```python
from build123d import *

# Parameters (mm, degrees)
SKETCH1_R           = 6.35
BOSS_EXTRUDE1_DEPTH = 31.75
BOSS_EXTRUDE2_DEPTH = 6.35
SKETCH3_R           = 6.35
CUT_EXTRUDE1_DEPTH  = 12.7
FILLET1_R           = 2.54


with BuildPart() as part:
    # Sketch1 → Boss-Extrude1 (new body)
    with BuildSketch(Plane.XY):
        with BuildLine():
            Line((6.565823388424392, 24.536706446302436), (50.800000000000004, 12.699999999999978))
            Line((50.800000000000004, 12.699999999999978), (50.800000000000004, -12.70000000000002))
            Line((50.800000000000004, -12.70000000000002), (6.565823388424392, -24.536706446302436))
            ThreePointArc((6.565823388424392, -24.536706446302436), (-25.400000000000006, 3.11e-15), (6.565823388424392, 24.536706446302436))
        make_face()
        Circle(SKETCH1_R, mode=Mode.SUBTRACT)
    boss_extrude1 = extrude(amount=BOSS_EXTRUDE1_DEPTH)

    # Sketch2 → Boss-Extrude2 (add)
    with BuildSketch(Plane.XY.offset(31.75)):
        with BuildLine():
            Line((50.80000000000001, -12.700000000000014), (50.800000000000004, 12.699999999999978))
            Line((50.800000000000004, 12.699999999999978), (28.910843041272116, 18.557360645652828))
            ThreePointArc((28.910843041272116, 18.557360645652825), (26.285427110394792, 9.443273439243344), (25.399999999999693, 0))
            ThreePointArc((25.399999999999693, 0), (26.285427110394785, -9.443273439243356), (28.910843041272116, -18.557360645652846))
            Line((28.910843041272113, -18.557360645652846), (50.80000000000001, -12.700000000000015))
        make_face()
    boss_extrude2 = extrude(amount=BOSS_EXTRUDE2_DEPTH)

    # Mirror1: Boss-Extrude1, Boss-Extrude2 across plane
    add(boss_extrude1.mirror(Plane.XY))
    add(boss_extrude2.mirror(Plane.XY))

    # Sketch3 → Cut-Extrude1 (cut)
    with BuildSketch(Plane(origin=(50.800000000000004, 0, 0), x_dir=(0, 0, -1), z_dir=(1, 0, 0))):
        Circle(SKETCH3_R)
    extrude(amount=-CUT_EXTRUDE1_DEPTH, mode=Mode.SUBTRACT)

    # Fillet1
    fillet1_edges = [part.edges().sort_by_distance(p)[0] for p in [
        (50.800000000000004, 12.699999999999978, 0),
        (50.80000000000001, -12.700000000000014, 0),
        (17.738333214848257, 21.54703354597763, 31.75),
        (-25.40000000000001, 5.33e-15, 31.75),
        (28.910843041272116, 18.557360645652828, 34.925),
        (28.910843041272116, -18.557360645652842, 34.925),
        (39.85542152063606, 15.628680322826403, 38.1),
        (25.3999999999997, -8.88e-15, 38.1),
        (39.855421520636064, -15.62868032282643, 38.1),
        (17.738333214848254, -21.54703354597764, 31.75),
        (50.80000000000001, -1.776e-14, 38.1),
        (17.738333214848254, -21.54703354597764, -31.75),
        (-25.40000000000001, 5.33e-15, -31.75),
        (17.738333214848257, 21.54703354597763, -31.75),
        (39.85542152063606, 15.628680322826403, -38.1),
        (28.910843041272116, 18.557360645652828, -34.925),
        (50.80000000000001, -1.776e-14, -38.1),
        (39.855421520636064, -15.62868032282643, -38.1),
        (25.3999999999997, -8.88e-15, -38.1),
        (28.910843041272116, -18.557360645652842, -34.925),
    ]]
    fillet(fillet1_edges, radius=FILLET1_R)


solid = part.part
```
CAD build for the part. Positions are in the model's coordinates, mm. A direction names the side the tool comes from. Round coordinates to 2 decimals unless told otherwise and drop trailing zeros. Loops run counter-clockwise (first coordinate to the right, second up) from the corner with the lowest first, then second, coordinate; pieces in that order, holes last. Notation, with made-up numbers: M 38.5,30.25 L 96.5,30.25 A16 ccw 96.5,55.25 Z; hole C 8,36.25 d3. An arc over 180 degrees is marked long. Return JSON: item names as keys, results as strings. Group by question number.
(1) Drop flat-ended pins along their axis: P1, Ø5, axis at y = 11.5, z = -12.5, coming from the -X side; P2, Ø1.5, axis at x = 29.5, z = 5, coming from the -Y side; P3, Ø10, axis at x = -7, y = 19.5, coming from the +Z side. Give the stop position or say it passes through.
(2) Saw through at B-B, the plane z = 0. List the corners of the cut face in (x, y), and give its area (3 significant figures).
(3) Tool access for faces 1 (the cylindrical face through (25.4, 0.2, 33.6)), 2 (the cylindrical face through (29.28, -17.73, -33.14)), 3 (the flat face through (38.1, 0, 0)), 4 (the cylindrical face through (29.28, 17.73, -33.14)): list every direction of +Z, -Z, +X, -X, +Y, -Y with a clear straight run to the whole face (end or side of a thin tool).
(4) Saw through at A-A, the plane x = 0. List the corners of the cut face in (y, z), and give its area (3 significant figures).
(5) Mould opens along Z. For faces 5 (the cylindrical face through (18.8, 20.5, -31)), 6 (the cylindrical face through (18.8, 20.5, 31)), 7 (the cylindrical face through (44.54, -6.2, 1.38)), 8 (the cylindrical face through (50.29, 12.28, 0.5)) say: +Z half, -Z half, draft (parallel to the pull), parting line (faces both ways), or undercut.
(6) Wall check: probe 1 along Y at (x, z) = (0, 7.5); probe 2 along X at (y, z) = (-0.5, 26.5); probe 3 along X at (y, z) = (-5, -21). Give the ranges that are in metal, low to high. Write a range as [from, to].
Answer list:
{
 "1": {"P1": "x = -23.75", "P2": "y = -18.6", "P3": "z = 31.75"},
 "2": {"outline": "M 6.57,-24.54 L 48.92,-13.2 A2.54 ccw 50.8,-10.75 L 50.8,-6.35 L 38.1,-6.35 L 38.1,6.35 L 50.8,6.35 L 50.8,10.75 A2.54 ccw 48.92,13.2 L 6.57,24.54 A25.4 ccw long Z; hole C 0,0 d12.7", "area": "2,700 mm2"},
 "3": {"face 1": "+Z, -X", "face 2": "-Z, -Y", "face 3": "+X", "face 4": "-Z, +Y"},
 "4": {"outline": "M -25.4,-29.21 A2.54 ccw -22.86,-31.75 L -6.35,-31.75 L -6.35,31.75 L -22.86,31.75 A2.54 ccw -25.4,29.21 Z; M 6.35,-31.75 L 22.86,-31.75 A2.54 ccw 25.4,-29.21 L 25.4,29.21 A2.54 ccw 22.86,31.75 L 6.35,31.75 Z", "area": "2,410 mm2"},
 "5": {"face 5": "-Z half", "face 6": "+Z half", "face 7": "undercut", "face 8": "draft"},
 "6": {"probe 1": "[-25.4, -6.35], [6.35, 25.4]", "probe 2": "[-25.4, -6.33], [6.33, 50.8]", "probe 3": "[-24.9, -3.91], [3.91, 50.8]"}
}
